Answer from the drawing. Dimensions are ordinates in mm from the lowest x, y and z of the part. Give positions to 0.01 mm unless a question says otherwise; leave off trailing zeros. Loops run counter-clockwise (first coordinate to the right, second up) from the corner with the lowest first, then second, coordinate; pieces in that order, holes last.
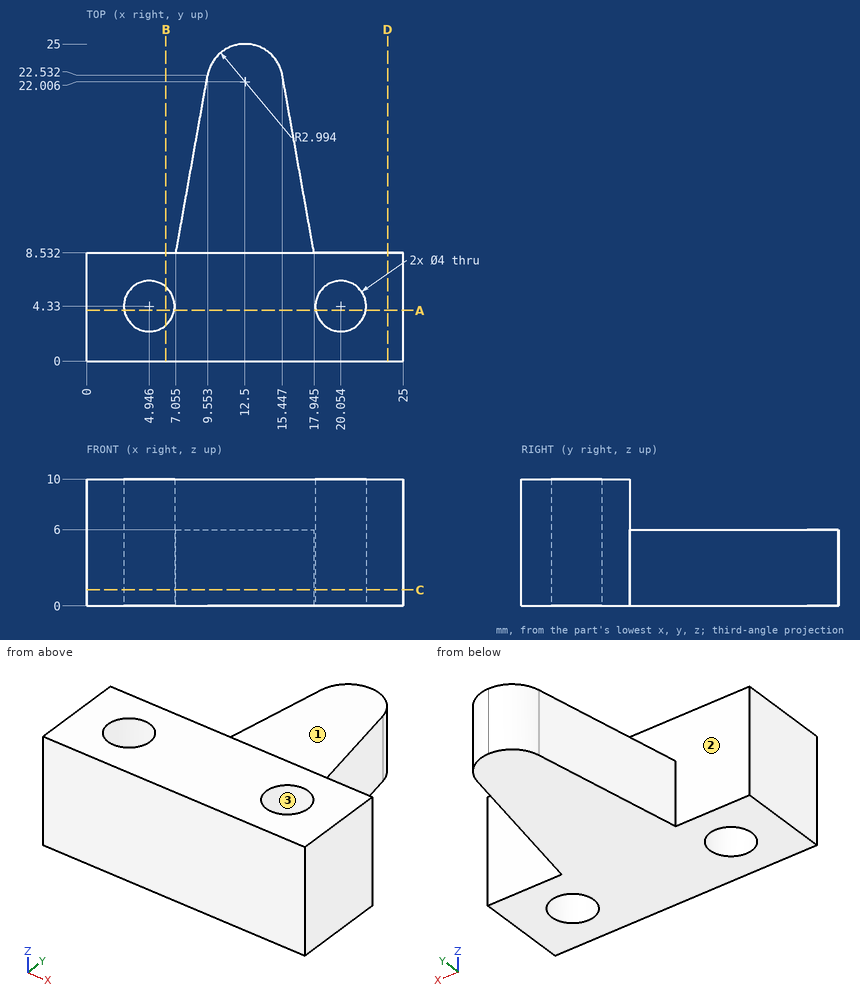
Item 1: Find section A-A, the plane y = 4. Write down the section's boundary in (x, z), plus the area to 3 significant figures.
Item 2: Find section B-B, the plane x = 6.25. Write down the section's boundary in (y, z).
Item 3: Find section D-D, the plane x = 23.75. Write down the section's boundary in (y, z).
Item 4: Find section C-C, the plane z = 1.25. Write down the section's boundary in (x, y) (1 decimal).
Item 5: Consider line 1 (Z direction, x = 15.5, y = 16.5); line 2 (X direction, y = 4, z = 7.75); line 3 (Y direction, x = 2.75, z = 7.75). Determine where each line is inside the solid, lowest interval first.
Item 6: A flat-ended cylindrical pin translates along its axis: pin 1 Ø2 at (y, z) = (13.5, 4) entering from +X. Find the tip coordinate at first contact, or state that the pin passes through.
Item 7: Determine the mould class of the marked faces 1, 2 and 3 for opening direction Y: released by +Y, released by -Y, zero draft, split by the parting line, or undercut.
Ans:
1. outline: (0, 0) - (2.97, 0) - (2.97, 10) - (0, 10) - close; (6.92, 0) - (18.08, 0) - (18.08, 10) - (6.92, 10) - close; (22.03, 0) - (25, 0) - (25, 10) - (22.03, 10) - close
1. area: 171 mm2
2. outline: (0, 0) - (2.81, 0) - (2.81, 10) - (0, 10) - close; (5.85, 0) - (8.53, 0) - (8.53, 10) - (5.85, 10) - close
3. outline: (0, 0) - (8.53, 0) - (8.53, 10) - (0, 10) - close
4. outline: (0, 0) - (25, 0) - (25, 8.5) - (17.9, 8.5) - (15.4, 22.5) arc R3 ccw to (12.5, 25) arc R3 ccw to (9.6, 22.5) - (7.1, 8.5) - (0, 8.5) - close; hole circle Ø4 at (4.9, 4.3); hole circle Ø4 at (20.1, 4.3)
5. line 1: z = 0 to 6
5. line 2: x = 0 to 2.97, 6.92 to 18.08, 22.03 to 25
5. line 3: y = 0 to 8.53
6. pin 1: stops at x = 17.24
7. face 1: zero draft
7. face 2: released by +Y
7. face 3: undercut
